```python
from build123d import *

# Parameters (mm, degrees)
EXTRUDE_THIN1_START = 10
EXTRUDE_THIN1_DEPTH = 100


with BuildPart() as part:
    # Sketch1 → Extrude-Thin1 (new body)
    with BuildSketch(Plane.XY.offset(EXTRUDE_THIN1_START)):
        with BuildLine():
            Line((264.897959184, -25), (-305.102040816, -25))
            ThreePointArc((-305.102040816, -25), (-330.102040816, 0), (-305.102040816, 25))
            Line((-305.102040816, 25), (264.897959184, 25))
            ThreePointArc((264.897959184, 25), (289.897959184, 0), (264.897959184, -25))
        make_face()
        with BuildLine():
            Line((264.897959184, -15), (-305.102040816, -15))
            ThreePointArc((-305.102040816, -15), (-320.102040816, 0), (-305.102040816, 15))
            Line((-305.102040816, 15), (264.897959184, 15))
            ThreePointArc((264.897959184, 15), (279.897959184, 0), (264.897959184, -15))
        make_face(mode=Mode.SUBTRACT)
    extrude(amount=EXTRUDE_THIN1_DEPTH)


solid = part.part
```
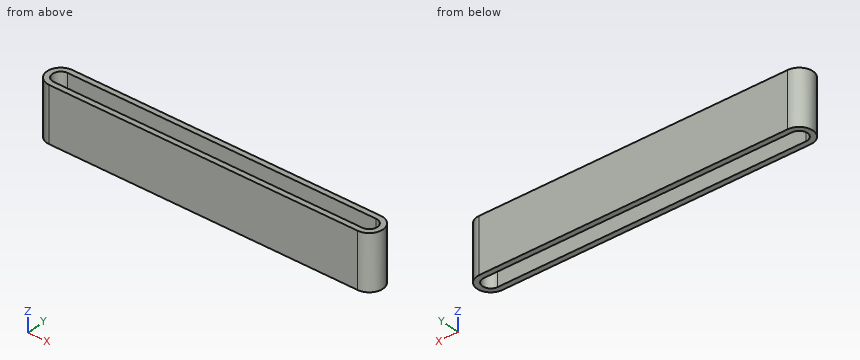
Verification items for the finished model (mm, model axes). Round coordinates to 2 decimals unless told otherwise and drop trailing zeros. Order: outer loops, then holes, each group sorted by start corner. A loop starts at its lowest first (then second) coordinate and runs counter-clockwise, first axis right, second up.
1) Depth check by flat-ended pin: pin 1 (1 mm diameter, centred on y = -15, z = 58, fed in from -X). Enter the tip coordinate at first touch or a pass-through.
Geometry says:
pin 1: stops at x = -325.47
2) Cross-section at B-B, the plane x = -140.5. Record the cut outline in (y, z).
Geometry says:
outline: (-25, 10) - (-15, 10) - (-15, 110) - (-25, 110) - close; (15, 10) - (25, 10) - (25, 110) - (15, 110) - close
3) Cross-section at C-C, the plane z = 84. Record the cut outline in (x, y), plus the area to 3 significant figures.
Geometry says:
outline: (-305.1, -25) - (264.9, -25) arc R25 ccw to (264.9, 25) - (-305.1, 25) arc R25 ccw to start; hole (-305.1, -15) - (264.9, -15) arc R15 ccw to (264.9, 15) - (-305.1, 15) arc R15 ccw to start
area: 12,700 mm2
4) Cross-section at A-A, the plane y = 0. Record the cut outline in (x, z).
Geometry says:
outline: (-330.1, 10) - (-320.1, 10) - (-320.1, 110) - (-330.1, 110) - close; (279.9, 10) - (289.9, 10) - (289.9, 110) - (279.9, 110) - close
5) Material ranges on line 1 (Y direction, x = 164, z = 68); line 2 (X direction, y = 7, z = 15); line 3 (X direction, y = -12.5, z = 45.5), recorded low to high.
Geometry says:
line 1: y = -25 to -15, 15 to 25
line 2: x = -329.1 to -318.37, 278.16 to 288.9
line 3: x = -326.75 to -313.39, 273.19 to 286.55
